```python
from build123d import *

# Parameters (mm, degrees)
EXTRUDE_1_DEPTH     = 8
FILLET_1_R          = 2
SKETCH_2_R          = 1.85
CUT_EXTRUDE_1_DEPTH = 7
CUT_EXTRUDE_START   = -8
SKETCH_3_R          = 1.85
CUT_EXTRUDE_2_DEPTH = 8
EXTRUDE_2_DEPTH     = 8
EXTRUDE_START       = 3
SKETCH_5_W          = 10
SKETCH_5_H          = 8
SKETCH_5_R          = 1.85
EXTRUDE_3_DEPTH     = 3
FILLET_2_R          = 3


with BuildPart() as part:
    # ｽｹｯﾁ1 → ﾎﾞｽ - 押し出し1 (new body)
    with BuildSketch(Plane.XY):
        Polygon((0, 0), (-10, 0), (-35, 23), (-35, 30), (0, 30), align=None)
        Polygon((-4, 26), (-4, 4), (-8.439899913, 4), (-32.352943391, 26), align=None, mode=Mode.SUBTRACT)
    extrude_1 = extrude(amount=EXTRUDE_1_DEPTH)

    # ﾐﾗｰ1: ﾎﾞｽ - 押し出し1 across plane
    add(extrude_1.mirror(Plane(origin=(0, 30, 8), x_dir=(0, 0, 1), z_dir=(-1, 0, 0))))

    # ﾌｨﾚｯﾄ1
    fillet_1_edges = [part.edges().sort_by_distance(p)[0] for p in [
        (-4, 26, 4),
        (-32.352943391, 26, 4),
        (-4, 4, 4),
        (4, 26, 4),
        (4, 4, 4),
        (32.352943391, 26, 4),
    ]]
    fillet(fillet_1_edges, radius=FILLET_1_R)

    # ｽｹｯﾁ2 → ｶｯﾄ - 押し出し1 (cut)
    with BuildSketch(Plane(origin=(0, 30, 0), x_dir=(1, 0, 0), z_dir=(0, 1, 0))):
        with Locations(Location((0, -4, 0), (0, 0, 270))):
            Circle(SKETCH_2_R)
        with Locations(Location((-30, -4, 0), (0, 0, 270))):
            Circle(SKETCH_2_R)
        with Locations(Location((30, -4, 0), (0, 0, 270))):
            Circle(SKETCH_2_R)
    extrude(amount=-CUT_EXTRUDE_1_DEPTH, mode=Mode.SUBTRACT)

    # ｽｹｯﾁ3 → ｶｯﾄ - 押し出し2 (cut)
    with BuildSketch(Plane(origin=(0, 0, 0), x_dir=(-1, 0, 0), z_dir=(0, -1, 0)).offset(CUT_EXTRUDE_START)):
        with Locations(Location((0, -4, 0), (0, 0, 270))):
            Circle(SKETCH_3_R)
    extrude(amount=CUT_EXTRUDE_2_DEPTH, mode=Mode.SUBTRACT)

    # ｽｹｯﾁ4 → ﾎﾞｽ - 押し出し2 (add)
    with BuildSketch(Plane(origin=(0, 0, 0), x_dir=(-1, 0, 0), z_dir=(0, 0, -1))):
        Polygon((5, 0), (5, -5), (10, 0), align=None)
        Polygon((-10, 0), (-5, 0), (-5, -5), align=None)
    extrude(amount=-EXTRUDE_2_DEPTH)

    # ｽｹｯﾁ5 → ﾎﾞｽ - 押し出し3 (add)
    # profile 1 of 2: a face of its own
    with BuildSketch(Plane(origin=(0, 30, 0), x_dir=(1, 0, 0), z_dir=(0, 1, 0)).offset(EXTRUDE_START)):
        with Locations((30, -4)):
            Rectangle(SKETCH_5_W, SKETCH_5_H)
        with Locations(Location((30, -4, 0), (0, 0, 270))):
            Circle(SKETCH_5_R, mode=Mode.SUBTRACT)
    # profile 2 of 2: a face of its own
    with BuildSketch(Plane(origin=(0, 30, 0), x_dir=(1, 0, 0), z_dir=(0, 1, 0)).offset(EXTRUDE_START)):
        with Locations((-30, -4)):
            Rectangle(SKETCH_5_W, SKETCH_5_H)
        with Locations(Location((-30, -4, 0), (0, 0, 270))):
            Circle(SKETCH_5_R, mode=Mode.SUBTRACT)
    extrude(amount=-EXTRUDE_3_DEPTH)

    # ﾌｨﾚｯﾄ2
    fillet_2_edges = [part.edges().sort_by_distance(p)[0] for p in [
        (-35, 28, 8),
        (35, 28, 8),
        (35, 28, 0),
        (-35, 28, 0),
    ]]
    fillet(fillet_2_edges, radius=FILLET_2_R)


solid = part.part
```
Can you work these out from the model? Positions are in its coordinate system, mm. A direction names the side the tool comes from. Round coordinates to 2 decimals unless told otherwise and drop trailing zeros. Loops run counter-clockwise (first coordinate to the right, second up) from the corner with the lowest first, then second, coordinate; pieces in that order, holes last. Notation, with made-up numbers: (6.5, -31.5) -> (13.5, -31.5) arc R19 cw to (13.5, -26.5) -> close; hole circle Ø8 at (-11.75, -13). An arc over 180 degrees is marked (long way). One line per item, written item: value. Start each with the question number.
1. For faces 1 (the flat face through (-25, 32, 4)), 2 (the cylindrical face through (-1.126, 26.549, 2.532)), 3 (the flat face through (-17, 26, 4)), 4 (the flat face through (0, 17, 0)), 5 (the flat face through (-1, 0, 6)), which set-ups out of +Z, -Z, +X, -X, +Y, -Y let a thin tool reach every point of the face, with its end or its side?
2. If we section it at A-A, the plane y = 28: Write out the boundary of the cut face in (x, z).
3. If we section it at C-C, the plane y = 16.5: Write out the boundary of the cut face in (x, z).
4. If we section it at B-B, the plane x = 0: Write out the boundary of the cut face in (y, z).
5. If we section it at D-D, the plane x = -22: Write out the boundary of the cut face in (y, z), then the cut area to 3 significant figures.
6. If I drill on probe 1 along X at (y, z) = (27.25, 4); probe 2 along X at (y, z) = (29, 5); probe 3 along X at (y, z) = (8, 2), over which ranges is the centre line in solid material (lowest first)?
7. For pin 1 (4.5 mm diameter, centred on x = 0, z = 4, fed in from -Y); pin 2 (0.7 mm diameter, centred on x = -7.5, z = 3, fed in from +Y); pin 3 (1.1 mm diameter, centred on x = 0.5, z = 3, fed in from +Y), each with a flat end and sliding along its axis, tell me the tip position at first contact or that it passes through.
8. If we mould it in two halves opening along Y, with no side actions, what happens to faces 6 (the flat face through (0, 30, 1)), 7 (the cylindrical face through (34.14, 28.13, 7.1)), 8 (the cylindrical face through (-4.57, 25.4, 4.06))? For each: pulls with the +Y half, pulls with the -Y half, needs draft (parallel to the pull), parting line crosses it, or undercut.
Calculated:
1. face 1: +Z, -Z, +Y
1. face 2: +Y
1. face 3: +Z, -Z
1. face 4: -Z, +X, -X, +Y, -Y
1. face 5: +Z, -Z, -Y
2. outline: (-35, 3) arc R3 ccw to (-32, 0) -> (32, 0) arc R3 ccw to (35, 3) -> (35, 5) arc R3 ccw to (32, 8) -> (-32, 8) arc R3 ccw to (-35, 5) -> close; hole circle Ø3.7 at (-30, 4); hole circle Ø3.7 at (0, 4); hole circle Ø3.7 at (30, 4)
3. outline: (-27.93, 0) -> (-22.03, 0) -> (-22.03, 8) -> (-27.93, 8) -> close; (-4, 0) -> (4, 0) -> (4, 8) -> (-4, 8) -> close; (22.03, 0) -> (27.93, 0) -> (27.93, 8) -> (22.03, 8) -> close
4. outline: (0, 0) -> (30, 0) -> (30, 2.15) -> (23, 2.15) -> (23, 5.85) -> (30, 5.85) -> (30, 8) -> (0, 8) -> (0, 5.85) -> (8, 5.85) -> (8, 2.15) -> (0, 2.15) -> close
5. outline: (11.04, 0) -> (16.48, 0) -> (16.48, 8) -> (11.04, 8) -> close; (26, 0) -> (30, 0) -> (30, 8) -> (26, 8) -> close
5. area: 75.5 mm²
6. probe 1: x = -35 to -31.85, -28.15 to -1.85, 1.85 to 28.15, 31.85 to 35
6. probe 2: x = -35 to -31.56, -28.44 to -1.56, 1.56 to 28.44, 31.56 to 35
6. probe 3: x = -18.7 to -12.79, -4 to 4, 12.79 to 18.7
7. pin 1: stops at y = 0
7. pin 2: stops at y = 30
7. pin 3: stops at y = 23
8. face 6: pulls with the +Y half
8. face 7: needs draft
8. face 8: undercut
